Input: part model. Units: mm. Frame: model coordinates. A direction names the side the tool comes from. Coordinates: 2 decimals unless noted, no trailing zeros. Write each loop counter-clockwise with the first axis right and the second up, starting at its lowest first coordinate (ties: lowest second). Pieces come first, ordered by that corner, then holes. Notation, with made-up numbers: (-28.5, 58) - (8.5, 58) arc R14 cw to (8.5, 73) - close; hole circle Ø11 at (66.25, -23.5). An arc over 180 degrees is marked (long way). Put each result on its own line as item: value. Start each with the question number.
1. Cut plane A-A, the plane x = 0. Return loops of the section in (y, z).
2. Cut plane B-B, the plane z = 7.25. Return loops of the section in (x, y), and give its area (3 significant figures).
3. Line query: line 1 (Y direction, x = 0, z = 5.75); line 2 (Y direction, x = -1, z = 2.25); line 3 (X direction, y = 0, z = 2). Output: solid intervals per line, ascending.
4. Cut plane D-D, the plane x = -10. Return loops of the section in (y, z), and give its area (3 significant figures).
5. Cut plane C-C, the plane y = 0. Return loops of the section in (x, z).
6. Pin query (flat end, axial travel): pin 1 (2.5 mm diameter, centred on y = 5.5, z = 3.5, fed in from +X); pin 2 (2 mm diameter, centred on x = 9, z = 2.5, fed in from -Y); pin 3 (2.5 mm diameter, centred on y = 13.5, z = 5, fed in from -X). Return the tip coordinate at first contact, or that it passes through.
7. Pull-direction query (Y, two-part tool) for faces 1 (the cylindrical face through (0, -5, 4)), 2 (the cylindrical face through (16.536, 1.048, 4.056)), 3 (the flat face through (10.415, -4.935, 3.944)), 4 (the flat face through (2, 6, 4)); classes: released by +Y, released by -Y, zero draft, split by the parting line, or undercut.
8. Access query for faces 5 (the flat face through (-5, 13, 4)), 6 (the flat face through (0, 18, 4)), 7 (the flat face through (-2, 6, 4)), 8 (the cylindrical face through (0, -10, 4)), 9 (the flat face through (5, 13, 4)). Directions: +Z, -Z, +X, -X, +Y, -Y. A direction counts if a zero-diameter tool reaches every point of the face in a straight line with its end or side. Return the directions, or none.
from build123d import *

# Parameters (mm, degrees)
SKETCH1_R           = 5
BOSS_EXTRUDE1_DEPTH = 8
BOSS_EXTRUDE2_DEPTH = 8
FILLET1_R           = 3
SKETCH3_W           = 4
SKETCH3_H           = 4.3
CUT_EXTRUDE1_DEPTH  = 26.720756349


with BuildPart() as part:
    # Sketch1 → Boss-Extrude1 (new body)
    with BuildSketch(Plane.XY):
        with BuildLine():
            Line((-5, 8.660254038), (-5, 18))
            Line((-5, 18), (5, 18))
            Line((5, 18), (5, 8.660254038))
            ThreePointArc((5, 8.660254038), (0, -10), (-5, 8.660254038))
        make_face()
        Circle(SKETCH1_R, mode=Mode.SUBTRACT)
    extrude(amount=BOSS_EXTRUDE1_DEPTH)

    # Sketch2 → Boss-Extrude2 (add)
    with BuildSketch(Plane(origin=(0, 0, 0), x_dir=(-1, 0, 0), z_dir=(0, 0, -1))):
        with BuildLine():
            Line((-5.711537543, -8.208430964), (-19.342239895, 1.275996517))
            Line((-19.342239895, 1.275996517), (-4.583721925, 8.887603351))
            ThreePointArc((-4.583721925, 8.887603351), (-9.978310939, 0.658263473), (-5.711537543, -8.208430964))
        make_face()
        with BuildLine():
            Line((5.711537543, -8.208430964), (19.342239895, 1.275996517))
            Line((19.342239895, 1.275996517), (4.583721925, 8.887603351))
            ThreePointArc((4.583721925, 8.887603351), (9.978310939, 0.658263473), (5.711537543, -8.208430964))
        make_face()
    extrude(amount=-BOSS_EXTRUDE2_DEPTH)

    # Fillet1
    fillet1_edges = [part.edges().sort_by_distance(p)[0] for p in [
        (19.342239895, 1.275996517, 4),
        (-19.342239895, 1.275996517, 4),
    ]]
    fillet(fillet1_edges, radius=FILLET1_R)

    # Sketch3 → Cut-Extrude1 (cut, through all)
    with BuildSketch(Plane(origin=(0, 0, 0), x_dir=(-1, 0, 0), z_dir=(0, 0, -1))):
        with Locations((0, 5.65)):
            Rectangle(SKETCH3_W, SKETCH3_H)
    extrude(amount=-CUT_EXTRUDE1_DEPTH, mode=Mode.SUBTRACT)


solid = part.part
Report:
1. outline: (-10, 0) - (-5, 0) - (-5, 8) - (-10, 8) - close; (7.8, 0) - (18, 0) - (18, 8) - (7.8, 8) - close
2. outline: (-15.25, -1.57) - (-5.71, -8.21) arc R10 ccw to (5.71, -8.21) - (15.25, -1.57) arc R3 ccw to (14.91, 3.56) - (5, 8.67) - (5, 18) - (-5, 18) - (-5, 8.67) - (-14.91, 3.56) arc R3 ccw to start; hole (-2, 4.58) arc R5 ccw (long way) to (2, 4.58) - (2, 7.8) - (-2, 7.8) - close
2. area: 423 mm^2
3. line 1: y = -10 to -5, 7.8 to 18
3. line 2: y = -9.95 to -4.9, 7.8 to 18
3. line 3: x = -16.4 to -5, 5 to 16.4
4. outline: (-5.22, 0) - (6.09, 0) - (6.09, 8) - (-5.22, 8) - close
4. area: 90.5 mm^2
5. outline: (-16.4, 0) - (-5, 0) - (-5, 8) - (-16.4, 8) - close; (5, 0) - (16.4, 0) - (16.4, 8) - (5, 8) - close
6. pin 1: stops at x = 13.58
6. pin 2: stops at y = -6.62
6. pin 3: stops at x = -5
7. face 1: undercut
7. face 2: split by the parting line
7. face 3: released by -Y
7. face 4: undercut
8. face 5: +Z, -Z, -X, +Y
8. face 6: +Z, -Z, +X, -X, +Y
8. face 7: +Z, -Z
8. face 8: +Z, -Z, -Y
8. face 9: +Z, -Z, +X, +Y
